```python
from build123d import *

# Parameters (mm, degrees)
SALIENTE_EXTRUIR1_DEPTH = 10
CROQUIS3_R              = 5
CROQUIS3_R_2            = 3.55
CROQUIS3_R_3            = 1.6
CORTAR_EXTRUIR1_DEPTH   = 11
CORTAR_EXTRUIR2_DEPTH   = 3.5
CROQUIS5_R              = 11.55
CORTAR_EXTRUIR3_DEPTH   = 5
CROQUIS8_W              = 15
CROQUIS8_H              = 29
SALIENTE_EXTRUIR2_DEPTH = 10
CROQUIS9_W              = 25
CROQUIS9_H              = 25
SALIENTE_EXTRUIR4_DEPTH = 10
CROQUIS13_R             = 12.5
SALIENTE_EXTRUIR5_DEPTH = 10
CROQUIS15_R             = 10.25
CORTAR_EXTRUIR5_DEPTH   = 20
CROQUIS16_R             = 1.6
CORTAR_EXTRUIR6_DEPTH   = 10
CROQUIS17_W             = 25
CROQUIS17_H             = 16.5
CROQUIS17_R             = 2
CROQUIS17_H_2           = 32.5
SALIENTE_EXTRUIR6_DEPTH = 10
REDONDEO1_R             = 1
CROQUIS18_W             = 5.6
CROQUIS18_H             = 12
CORTAR_EXTRUIR7_DEPTH   = 3
CORTAR_EXTRUIR10_START  = 60
CROQUIS19_R             = 1.6
CORTAR_EXTRUIR10_DEPTH  = 11.0000001


with BuildPart() as part:
    # Croquis1 → Saliente-Extruir1 (new body)
    with BuildSketch(Plane(origin=(0, 0, 0), x_dir=(1, 0, 0), z_dir=(0, 1, 0))):
        Polygon((-45, -22.5), (45, -22.5), (45, 22.5), (0, 22.5), (-45, 22.5), align=None)
    extrude(amount=SALIENTE_EXTRUIR1_DEPTH)

    # Croquis3 → Cortar-Extruir1 (cut, through all)
    with BuildSketch(Plane(origin=(0, 10, 0), x_dir=(1, 0, 0), z_dir=(0, 1, 0))):
        with Locations((-30, -2.5)):
            Circle(CROQUIS3_R)
        with Locations((30, -2.5)):
            Circle(CROQUIS3_R_2)
        with Locations((-38.25, -2.5)):
            Circle(CROQUIS3_R_3)
        with Locations((-21.75, -2.5)):
            Circle(CROQUIS3_R_3)
    extrude(amount=-CORTAR_EXTRUIR1_DEPTH, mode=Mode.SUBTRACT)

    # Croquis4 → Cortar-Extruir2 (cut)
    with BuildSketch(Plane(origin=(0, 10, 0), x_dir=(1, 0, 0), z_dir=(0, 1, 0))):
        Polygon((-38.25, 0.733161507), (-41.05, -0.883419246), (-41.05, -4.116580754), (-38.25, -5.733161507), (-35.45, -4.116580754), (-35.45, -0.883419246), align=None)
        Polygon((-21.75, 0.733161507), (-24.55, -0.883419246), (-24.55, -4.116580754), (-21.75, -5.733161507), (-18.95, -4.116580754), (-18.95, -0.883419246), align=None)
    extrude(amount=-CORTAR_EXTRUIR2_DEPTH, mode=Mode.SUBTRACT)

    # Croquis5 → Cortar-Extruir3 (cut)
    with BuildSketch(Plane.XZ):
        with Locations((-30, 2.5)):
            Circle(CROQUIS5_R)
    extrude(amount=-CORTAR_EXTRUIR3_DEPTH, mode=Mode.SUBTRACT)

    # Croquis8 → Saliente-Extruir2 (add)
    with BuildSketch(Plane(origin=(0, 10, 0), x_dir=(1, 0, 0), z_dir=(0, 1, 0))):
        with Locations((-37.5, 37)):
            Rectangle(CROQUIS8_W, CROQUIS8_H)
        with BuildLine():
            Line((-36.35, 39.5), (-36.35, 37.5))
            ThreePointArc((-36.35, 37.5), (-38, 35.85), (-39.65, 37.5))
            Line((-39.65, 37.5), (-39.65, 39.5))
            ThreePointArc((-39.65, 39.5), (-38, 41.15), (-36.35, 39.5))
        make_face(mode=Mode.SUBTRACT)
        with Locations((37.5, 37)):
            Rectangle(CROQUIS8_W, CROQUIS8_H)
        with BuildLine():
            Line((39.65, 46.5), (39.65, 44.5))
            ThreePointArc((39.65, 44.5), (38, 42.85), (36.35, 44.5))
            Line((36.35, 44.5), (36.35, 46.5))
            ThreePointArc((36.35, 46.5), (38, 48.15), (39.65, 46.5))
        make_face(mode=Mode.SUBTRACT)
    extrude(amount=-SALIENTE_EXTRUIR2_DEPTH)

    # Croquis9 → Saliente-Extruir4 (add)
    with BuildSketch(Plane(origin=(0, 0, 0), x_dir=(1, 0, 0), z_dir=(0, 1, 0))):
        with Locations((-57.5, 22.5)):
            Rectangle(CROQUIS9_W, CROQUIS9_H)
        with Locations((57.5, 22.5)):
            Rectangle(CROQUIS9_W, CROQUIS9_H)
    extrude(amount=SALIENTE_EXTRUIR4_DEPTH)

    # Croquis13 → Saliente-Extruir5 (add)
    with BuildSketch(Plane(origin=(0, 10, 0), x_dir=(1, 0, 0), z_dir=(0, 1, 0))):
        with Locations((-57.5, 22.5)):
            Circle(CROQUIS13_R)
        with Locations((57.5, 22.5)):
            Circle(CROQUIS13_R)
    extrude(amount=SALIENTE_EXTRUIR5_DEPTH)

    # Croquis15 → Cortar-Extruir5 (cut)
    with BuildSketch(Plane(origin=(0, 20, 0), x_dir=(1, 0, 0), z_dir=(0, 1, 0))):
        with Locations((-57.5, 22.5)):
            Circle(CROQUIS15_R)
        with Locations((57.5, 22.5)):
            Circle(CROQUIS15_R)
    extrude(amount=-CORTAR_EXTRUIR5_DEPTH, mode=Mode.SUBTRACT)

    # Croquis16 → Cortar-Extruir6 (cut)
    with BuildSketch(Plane(origin=(0, 0, -35), x_dir=(-1, 0, 0), z_dir=(0, 0, -1))):
        with Locations((-57.5, 15)):
            Circle(CROQUIS16_R)
        with Locations((57.5, 15)):
            Circle(CROQUIS16_R)
    extrude(amount=-CORTAR_EXTRUIR6_DEPTH, mode=Mode.SUBTRACT)

    # Croquis17 → Saliente-Extruir6 (add)
    with BuildSketch(Plane(origin=(0, 0, 0), x_dir=(1, 0, 0), z_dir=(0, 1, 0))):
        with Locations((57.5, 43.25)):
            Rectangle(CROQUIS17_W, CROQUIS17_H)
        with Locations((60, 41.5)):
            Circle(CROQUIS17_R, mode=Mode.SUBTRACT)
        with Locations((57.5, -6.25)):
            Rectangle(CROQUIS17_W, CROQUIS17_H_2)
        with Locations((60, -12.5)):
            Circle(CROQUIS17_R, mode=Mode.SUBTRACT)
        with Locations((-57.5, 43.25)):
            Rectangle(CROQUIS17_W, CROQUIS17_H)
        with Locations((-60, 41.5)):
            Circle(CROQUIS17_R, mode=Mode.SUBTRACT)
        with Locations((-57.5, -6.25)):
            Rectangle(CROQUIS17_W, CROQUIS17_H_2)
        with Locations((-60, -12.5)):
            Circle(CROQUIS17_R, mode=Mode.SUBTRACT)
    extrude(amount=SALIENTE_EXTRUIR6_DEPTH)

    # Redondeo1
    redondeo1_edges = [part.edges().sort_by_distance(p)[0] for p in [
        (-30, 5, -22.5),
        (-30, 5, -51.5),
        (-70, 5, -51.5),
        (-70, 5, 22.5),
        (70, 5, -51.5),
        (70, 5, 22.5),
        (30, 5, -22.5),
        (30, 5, -51.5),
    ]]
    fillet(redondeo1_edges, radius=REDONDEO1_R)

    # Croquis18 → Cortar-Extruir7 (cut)
    with BuildSketch(Plane.XZ):
        with Locations((-38, -38.5)):
            Rectangle(CROQUIS18_W, CROQUIS18_H)
        with Locations((38, -45.5)):
            Rectangle(CROQUIS18_W, CROQUIS18_H)
    extrude(amount=-CORTAR_EXTRUIR7_DEPTH, mode=Mode.SUBTRACT)

    # Croquis19 → Cortar-Extruir10 (cut, through all)
    with BuildSketch(Plane(origin=(0, 0, 0), x_dir=(0, 0, -1), z_dir=(1, 0, 0)).offset(CORTAR_EXTRUIR10_START)):
        with Locations((22.5, 15)):
            Circle(CROQUIS19_R)
    cortar_extruir10 = extrude(amount=CORTAR_EXTRUIR10_DEPTH, mode=Mode.SUBTRACT)

    # Simetría1: Cortar-Extruir10 across plane
    add(cortar_extruir10.mirror(Plane(origin=(0, 0, 0), x_dir=(0, 0, 1), z_dir=(1, 0, 0))), mode=Mode.SUBTRACT)


solid = part.part
```
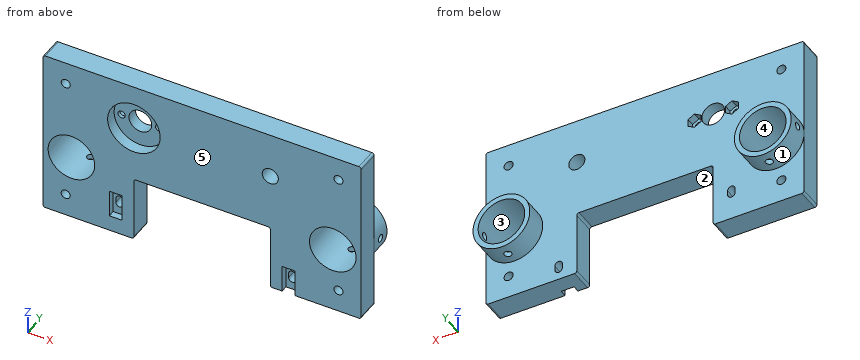
Geometry check sheet. Reference: the model listing, model coordinates, mm. Face numbers are marked on the shaded views. A direction names the side the tool comes from. Coordinates: 2 decimals unless noted, no trailing zeros. Write each loop counter-clockwise with the first axis right and the second up, starting at its lowest first coordinate (ties: lowest second). Pieces come first, ordered by that corner, then holes. Notation, with made-up numbers: M 49,80 L 86,80 A29 ccw 86,114 Z; hole C 16,48.25 d4. An arc over 180 degrees is marked long. Use one line per item in the form item = value. Start each with the question number.
1) Section check D-D on x = 6.5. Enter the section's corners in (y, z), and give its area (3 significant figures).
2) Release check for a two-part mould opening along X. For the marked faces 4 and 5 record: pulls with the +X half, pulls with the -X half, needs draft (parallel to the pull), parting line crosses it, or undercut.
3) Section check C-C on z = -18.5. Enter the section's corners in (x, y), and give its area (3 significant figures).
4) Section check B-B on z = -27.5. Enter the section's corners in (x, y).
5) Thickness scan on probe 1 along X at (y, z) = (5.65, 2.5); probe 2 along X at (y, z) = (7.75, 12.5); probe 3 along X at (y, z) = (2, -33.5). Record the ranges inside material, lowest first. Write a range as from..to.
6) Section check A-A on x = 38. Enter the section's corners in (y, z), and give its area (3 significant figures).
7) Set-up check for the marked faces 1, 2 and 3: record each of +Z, -Z, +X, -X, +Y, -Y from which the full face is reachable in a straight line by a thin tool's end or side.
8) Go/stop test with flat-tipped pins: pin 1 Ø3 at (x, y) = (12, 6.5) entering from -Z; pin 2 Ø5 at (x, y) = (57.5, 15) entering from +Z; pin 3 Ø5 at (x, z) = (-49, -19.5) entering from +Y; pin 4 Ø3.5 at (x, z) = (-60, 12.5) entering from +Y. Record where each tip stops, or that it passes through.
Responses:
q1.outline = M 0,-22.5 L 10,-22.5 L 10,22.5 L 0,22.5 Z
q1.area = 450 mm2
q2.face_4 = undercut
q2.face_5 = needs draft
q3.outline = M -70,0 L -66.94,0 L -66.94,20 L -69.34,20 L -69.34,10 L -70,10 Z; M -48.06,0 L 48.06,0 L 48.06,20 L 45.66,20 L 45.66,10 L -45.66,10 L -45.66,20 L -48.06,20 Z; M 66.94,0 L 70,0 L 70,10 L 69.34,10 L 69.34,20 L 66.94,20 Z
q3.area = 1,120 mm2
q4.outline = M -70,0 L -66.45,0 L -66.45,20 L -68.96,20 L -68.96,10 L -70,10 Z; M -48.55,0 L -30,0 L -30,10 L -46.04,10 L -46.04,20 L -48.55,20 Z; M 30,0 L 48.55,0 L 48.55,20 L 46.04,20 L 46.04,10 L 30,10 Z; M 66.45,0 L 70,0 L 70,10 L 68.96,10 L 68.96,20 L 66.45,20 Z
q5.probe_1 = -70..-39.85, -36.65..-35, -25..-23.35, -20.15..26.45, 33.55..70
q5.probe_2 = -70..-62, -58..58, 62..70
q5.probe_3 = -70..-40.8, -35.2..-30, 30..70
q6.outline = M 0,-39.5 L 3,-39.5 L 3,-42.85 L 10,-42.85 L 10,22.5 L 0,22.5 Z; M 3,-51.5 L 10,-51.5 L 10,-48.15 L 3,-48.15 Z
q6.area = 667 mm2
q7.face_1 = +Y
q7.face_2 = -Z, +Y, -Y
q7.face_3 = +Y, -Y
q8.pin_1 = -22.5
q8.pin_2 = -10
q8.pin_3 = 20
q8.pin_4 = through
